```python
from build123d import *

# Parameters (mm, degrees)
SKETCH2_W           = 108
SKETCH2_H           = 70
SKETCH2_R           = 2.25
SKETCH2_W_2         = 8
SKETCH2_H_2         = 14.5
BOSS_EXTRUDE1_DEPTH = 3
SKETCH5_R           = 3.5635
SKETCH5_R_2         = 1.6865
BOSS_EXTRUDE2_DEPTH = 17
SKETCH6_R           = 1.6865
BOSS_EXTRUDE3_DEPTH = 20.6
SKETCH7_W           = 108
SKETCH7_H           = 70
SKETCH7_W_2         = 102
SKETCH7_H_2         = 64
BOSS_EXTRUDE4_DEPTH = 17.05
SKETCH8_W           = 89.4
SKETCH8_H           = 3
CUT_EXTRUDE1_DEPTH  = 9.5
SKETCH9_W           = 46
SKETCH9_H           = 3
CUT_EXTRUDE2_DEPTH  = 17
SKETCH10_W          = 54.9
SKETCH10_H          = 7.1
CUT_EXTRUDE3_DEPTH  = 78.578234855
SKETCH11_R          = 3.496784868
CUT_EXTRUDE4_DEPTH  = 115.723751218
CUT_EXTRUDE5_START  = -1
SKETCH12_W          = 14.400869084
SKETCH12_H          = 17.05
SKETCH12_R          = 3.496784868
CUT_EXTRUDE5_DEPTH  = 1
SKETCH14_R          = 1.5
SKETCH14_W          = 18.05
SKETCH14_H          = 3.8
SKETCH14_H_2        = 5.5
CUT_EXTRUDE7_DEPTH  = 78.578234855
SKETCH15_R          = 2.5
CUT_EXTRUDE10_DEPTH = 1
SKETCH17_W          = 12
SKETCH17_H          = 18
SKETCH17_R          = 3.25
BOSS_EXTRUDE5_DEPTH = 20.05
FILLET1_R           = 2


with BuildPart() as part:
    # Sketch2 → Boss-Extrude1 (new body)
    # profile 1 of 2: a face of its own
    with BuildSketch(Plane(origin=(0, 0, 0), x_dir=(1, 0, 0), z_dir=(0, 1, 0))):
        with Locations((-7.231065886, 6.378485879)):
            Rectangle(SKETCH2_W, SKETCH2_H)
        with Locations(Location((-19.731065886, 20.878485879, 0), (0, 0, 270))):
            Circle(SKETCH2_R, mode=Mode.SUBTRACT)
        with Locations(Location((-19.731065886, 12.878485879, 0), (0, 0, 270))):
            Circle(SKETCH2_R, mode=Mode.SUBTRACT)
        with Locations(Location((-19.731065886, 4.878485879, 0), (0, 0, 270))):
            Circle(SKETCH2_R, mode=Mode.SUBTRACT)
        with Locations(Location((-9.731065886, 20.878485879, 0), (0, 0, 270))):
            Circle(SKETCH2_R, mode=Mode.SUBTRACT)
        with Locations(Location((-9.731065886, 12.878485879, 0), (0, 0, 270))):
            Circle(SKETCH2_R, mode=Mode.SUBTRACT)
        with Locations(Location((-9.731065886, 4.878485879, 0), (0, 0, 270))):
            Circle(SKETCH2_R, mode=Mode.SUBTRACT)
        with Locations(Location((20.268934114, 20.878485879, 0), (0, 0, 270))):
            Circle(SKETCH2_R, mode=Mode.SUBTRACT)
        with Locations((20.268934114, 12.878485879)):
            Circle(SKETCH2_R, mode=Mode.SUBTRACT)
        with Locations(Location((0.268934114, 20.878485879, 0), (0, 0, 270))):
            Circle(SKETCH2_R, mode=Mode.SUBTRACT)
        with Locations(Location((10.268934114, 20.878485879, 0), (0, 0, 270))):
            Circle(SKETCH2_R, mode=Mode.SUBTRACT)
        with Locations(Location((0.268934114, 12.878485879, 0), (0, 0, 270))):
            Circle(SKETCH2_R, mode=Mode.SUBTRACT)
        with Locations(Location((10.268934114, 12.878485879, 0), (0, 0, 270))):
            Circle(SKETCH2_R, mode=Mode.SUBTRACT)
        with Locations(Location((0.268934114, 4.878485879, 0), (0, 0, 270))):
            Circle(SKETCH2_R, mode=Mode.SUBTRACT)
        with Locations(Location((10.268934114, 4.878485879, 0), (0, 0, 270))):
            Circle(SKETCH2_R, mode=Mode.SUBTRACT)
        with Locations(Location((20.268934114, 4.878485879, 0), (0, 0, 270))):
            Circle(SKETCH2_R, mode=Mode.SUBTRACT)
        with Locations((-21.231065886, -7.871514121)):
            Rectangle(SKETCH2_W_2, SKETCH2_H_2, mode=Mode.SUBTRACT)
    # profile 2 of 2: a face of its own
    with BuildSketch(Plane(origin=(0, 0, 0), x_dir=(1, 0, 0), z_dir=(0, 1, 0))):
        with Locations((20.268934114, 12.878485879)):
            Circle(SKETCH2_R)
    extrude(amount=BOSS_EXTRUDE1_DEPTH)

    # Sketch5 → Boss-Extrude2 (add)
    # profile 1 of 4: a face of its own
    with BuildSketch(Plane(origin=(0, 0, 0), x_dir=(-1, 0, 0), z_dir=(0, -1, 0))):
        with Locations(Location((37.231065886, 32.378485879, 0), (0, 0, 270))):
            Circle(SKETCH5_R)
        with Locations(Location((37.231065886, 32.378485879, 0), (0, 0, 90))):
            Circle(SKETCH5_R_2, mode=Mode.SUBTRACT)
    # profile 2 of 4: a face of its own
    with BuildSketch(Plane(origin=(0, 0, 0), x_dir=(-1, 0, 0), z_dir=(0, -1, 0))):
        with Locations(Location((-37.768934114, 32.378485879, 0), (0, 0, 270))):
            Circle(SKETCH5_R)
        with Locations(Location((-37.768934114, 32.378485879, 0), (0, 0, 90))):
            Circle(SKETCH5_R_2, mode=Mode.SUBTRACT)
    # profile 3 of 4: a face of its own
    with BuildSketch(Plane(origin=(0, 0, 0), x_dir=(-1, 0, 0), z_dir=(0, -1, 0))):
        with Locations(Location((-37.768934114, -6.621514121, 0), (0, 0, 270))):
            Circle(SKETCH5_R)
        with Locations(Location((-37.768934114, -6.621514121, 0), (0, 0, 90))):
            Circle(SKETCH5_R_2, mode=Mode.SUBTRACT)
    # profile 4 of 4: a face of its own
    with BuildSketch(Plane(origin=(0, 0, 0), x_dir=(-1, 0, 0), z_dir=(0, -1, 0))):
        with Locations(Location((37.231065886, -6.621514121, 0), (0, 0, 270))):
            Circle(SKETCH5_R)
        with Locations(Location((37.231065886, -6.621514121, 0), (0, 0, 90))):
            Circle(SKETCH5_R_2, mode=Mode.SUBTRACT)
    extrude(amount=BOSS_EXTRUDE2_DEPTH)

    # Sketch6 → Boss-Extrude3 (add)
    with BuildSketch(Plane(origin=(0, 0, 0), x_dir=(-1, 0, 0), z_dir=(0, -1, 0))):
        with Locations(Location((37.231065886, 32.378485879, 0), (0, 0, 270))):
            Circle(SKETCH6_R)
        with Locations(Location((-37.768934114, 32.378485879, 0), (0, 0, 270))):
            Circle(SKETCH6_R)
        with Locations(Location((-37.768934114, -6.621514121, 0), (0, 0, 270))):
            Circle(SKETCH6_R)
        with Locations(Location((37.231065886, -6.621514121, 0), (0, 0, 270))):
            Circle(SKETCH6_R)
    extrude(amount=BOSS_EXTRUDE3_DEPTH)

    # Sketch7 → Boss-Extrude4 (add)
    with BuildSketch(Plane(origin=(0, 0, 0), x_dir=(-1, 0, 0), z_dir=(0, -1, 0))):
        with Locations((7.231065886, 6.378485879)):
            Rectangle(SKETCH7_W, SKETCH7_H)
        with Locations((7.231065886, 6.378485879)):
            Rectangle(SKETCH7_W_2, SKETCH7_H_2, mode=Mode.SUBTRACT)
    extrude(amount=BOSS_EXTRUDE4_DEPTH)

    # Sketch8 → Cut-Extrude1 (cut)
    with BuildSketch(Plane.XZ.offset(17.05)):
        with Locations((-7.131065886, 27.121514121)):
            Rectangle(SKETCH8_W, SKETCH8_H)
    extrude(amount=-CUT_EXTRUDE1_DEPTH, mode=Mode.SUBTRACT)

    # Sketch9 → Cut-Extrude2 (cut)
    with BuildSketch(Plane.XZ.offset(17.05)):
        with Locations((-8.231065886, 27.121514121)):
            Rectangle(SKETCH9_W, SKETCH9_H)
    extrude(amount=-CUT_EXTRUDE2_DEPTH, mode=Mode.SUBTRACT)

    # Sketch10 → Cut-Extrude3 (cut, through all)
    with BuildSketch(Plane(origin=(0, 3, 0), x_dir=(1, 0, 0), z_dir=(0, 1, 0))):
        with Locations((5.818934114, 32.828485879)):
            Rectangle(SKETCH10_W, SKETCH10_H)
    extrude(amount=-CUT_EXTRUDE3_DEPTH, mode=Mode.SUBTRACT)

    # Sketch11 → Cut-Extrude4 (cut, through all)
    with BuildSketch(Plane(origin=(-58.231065886, 0, 0), x_dir=(0, 0, -1), z_dir=(1, 0, 0))):
        with Locations((-8.621514121, -8.525)):
            Circle(SKETCH11_R)
        with Locations(Location((21.378485879, -8.525, 0), (0, 0, 180))):
            Circle(SKETCH11_R)
    extrude(amount=-CUT_EXTRUDE4_DEPTH, mode=Mode.SUBTRACT)

    # Sketch12 → Cut-Extrude5 (cut)
    # profile 1 of 2: a face of its own
    with BuildSketch(Plane.ZY.offset(61.231065886).offset(CUT_EXTRUDE5_START)):
        with Locations((-22.578920421, -8.525)):
            Rectangle(SKETCH12_W, SKETCH12_H)
        with Locations((-21.378485879, -8.525)):
            Circle(SKETCH12_R, mode=Mode.SUBTRACT)
    # profile 2 of 2: a face of its own
    with BuildSketch(Plane.ZY.offset(61.231065886).offset(CUT_EXTRUDE5_START)):
        with Locations((9.821948663, -8.525)):
            Rectangle(SKETCH12_W, SKETCH12_H)
        with Locations(Location((8.621514121, -8.525, 0), (0, 0, 180))):
            Circle(SKETCH12_R, mode=Mode.SUBTRACT)
    extrude(amount=CUT_EXTRUDE5_DEPTH, mode=Mode.SUBTRACT)

    # Sketch14 → Cut-Extrude7 (cut, through all)
    with BuildSketch(Plane(origin=(0, 3, 0), x_dir=(1, 0, 0), z_dir=(0, 1, 0))):
        with Locations(Location((31.278934114, -19.931514121, 0), (0, 0, 270))):
            Circle(SKETCH14_R)
        with Locations(Location((17.308934114, -19.931514121, 0), (0, 0, 270))):
            Circle(SKETCH14_R)
        with Locations((24.293934114, 13.088485879)):
            Rectangle(SKETCH14_W, SKETCH14_H)
        with Locations((24.293934114, -13.371514121)):
            Rectangle(SKETCH14_W, SKETCH14_H_2)
    extrude(amount=-CUT_EXTRUDE7_DEPTH, mode=Mode.SUBTRACT)

    # Sketch15 → Cut-Extrude10 (cut)
    with BuildSketch(Plane.XZ):
        with Locations(Location((17.308934114, 19.931514121, 0), (0, 0, 270))):
            Circle(SKETCH15_R)
        with Locations(Location((31.278934114, 19.931514121, 0), (0, 0, 270))):
            Circle(SKETCH15_R)
    extrude(amount=-CUT_EXTRUDE10_DEPTH, mode=Mode.SUBTRACT)

    # Sketch17 → Boss-Extrude5 (add)
    # profile 1 of 2: a face of its own
    with BuildSketch(Plane.XZ.offset(17.05)):
        with Locations((-67.231065886, -6.378485879)):
            Rectangle(SKETCH17_W, SKETCH17_H)
        with Locations(Location((-65.731065886, -6.378485879, 0), (0, 0, 270))):
            Circle(SKETCH17_R, mode=Mode.SUBTRACT)
    # profile 2 of 2: a face of its own
    with BuildSketch(Plane.XZ.offset(17.05)):
        with Locations((52.768934114, -6.378485879)):
            Rectangle(SKETCH17_W, SKETCH17_H)
        with Locations(Location((51.268934114, -6.378485879, 0), (0, 0, 270))):
            Circle(SKETCH17_R, mode=Mode.SUBTRACT)
    extrude(amount=-BOSS_EXTRUDE5_DEPTH)

    # Fillet1
    fillet1_edges = [part.edges().sort_by_distance(p)[0] for p in [
        (-73.231065886, -7.025, -15.378485879),
        (-73.231065886, -7.025, 2.621514121),
        (58.768934114, -7.025, -15.378485879),
        (58.768934114, -7.025, 2.621514121),
    ]]
    fillet(fillet1_edges, radius=FILLET1_R)


solid = part.part
```
Work out the finished part from the listing and answer in its coordinate system (mm). A direction names the side the tool comes from. Give positions to 0.01 mm unless a question says otherwise; leave off trailing zeros. Order: outer loops, then holes, each group sorted by start corner. A loop starts at its lowest first (then second) coordinate and runs counter-clockwise, first axis right, second up.
1. For faces 1 (the flat face through (-60.231, -8, -26)), 2 (the flat face through (39, -17, -31)), 3 (the flat face through (-9, -0.05, 27)), 4 (the flat face through (24, 2, 16.122)), determine the directions among +Z, -Z, +X, -X, +Y, -Y from which every point of the face is accessible in a straight line to the end or side of a thin tool.
Result sheet:
face 1: -X, -Y
face 2: -Y
face 3: +Z, -Y
face 4: +Y, -Y
2. Section B-B, the plane y = -13.5 is taken. Give the number of separate pieces and of enclosed holes in the cut face, and give its area (3 significant figures).
Result sheet:
separate pieces: 5
enclosed holes: 2
area: 1,260 mm2
3. The mould has two halves that part along Z. Classify faces 5 (the flat face through (46.769, -7, 16)), 6 (the flat face through (-21, 1, 15.122)): released by +Z, released by -Z, zero draft, split by the parting line, or undercut.
Result sheet:
face 5: zero draft
face 6: undercut
4. Section A-A, the plane x = 27 is taken. Determine the outline of the cut face in (y, z), and give its area (3 significant figures).
Result sheet:
outline: (-17.05, -41.38) - (3, -41.38) - (3, -36.38) - (0, -36.38) - (0, -38.38) - (-17.05, -38.38) - close; (-7.55, 25.62) - (0, 25.62) - (0, 16.12) - (3, 16.12) - (3, 28.62) - (-7.55, 28.62) - close; (0, -29.28) - (3, -29.28) - (3, -14.99) - (0, -14.99) - close; (0, -11.19) - (3, -11.19) - (3, 10.62) - (0, 10.62) - close
area: 235 mm2
5. Each of these flat-tipped pins is pushed along its axis until it touches: P1, Ø1, axis at x = -1.5, y = -1, coming from the +Z side; P2, Ø8, axis at y = -5, z = 17.5, coming from the +X side; P3, Ø2, axis at x = 11.5, z = -32, coming from the +Y side; P4, Ø1.5, axis at y = -12, z = 27, coming from the -X side. Where does it stop, or does it pass through?
Result sheet:
P1: stops at z = -38.38
P2: stops at x = 46.77
P3: passes through
P4: stops at x = -61.23
6. Straight lines are drawn through the part: L1, parallel to Z at x = -37, y = -5; L2, parallel to Z at x = -61, y = -11.5; L3, parallel to Z at x = -55.5, y = -7.5. For each, find the intervals that lie inside material, in ascending order.
Result sheet:
L1: z = -41.38 to -38.38, -35.93 to -28.82, 3.07 to 10.18, 25.62 to 28.62
L2: z = -41.38 to -29.78, -15.38 to 2.62, 17.02 to 28.62
L3: z = -41.38 to -38.38, 25.62 to 28.62
7. Section C-C, the plane x = -48.5 is taken. Determine the outline of the cut face in (y, z).
Result sheet:
outline: (-17.05, -41.38) - (3, -41.38) - (3, 28.62) - (-7.55, 28.62) - (-7.55, 25.62) - (0, 25.62) - (0, -38.38) - (-17.05, -38.38) - close
